Could you check a few things on this model? Use its own coordinates, in mm. A direction names the side the tool comes from. Coordinates: 2 decimals unless noted, no trailing zeros. Write each loop counter-clockwise with the first axis right and the second up, starting at its lowest first coordinate (ties: lowest second). Pieces come first, ordered by that corner, then holes. Notation, with made-up numbers: (58, 2.25) - (89, 2.25) arc R13 ccw to (89, 7.25) - close; hole circle Ø1 at (35.5, 60.25). An arc over 180 degrees is marked (long way). Answer as a JSON object with one key per item and string values. Group by question number.
1) If we section it at A-A (y = 7.62): Write out the boundary of the cut face in (x, z), plus the area to 3 significant figures.
2) If we section it at D-D (x = 13.25): Write out the boundary of the cut face in (y, z), plus the area to 3 significant figures.
3) We'd pull the mould along X, two halves only. Please class faces 1 (the cylindrical face through (5.854, 18.371, -19.108)), 2 (the flat face through (13.26, 7.51, -21.65)), 3 (the flat face through (-8, 8, -8)): released by +X, released by -X, zero draft, split by the parting line, or undercut.
4) If we section it at B-B (x = 6.35): Write out the boundary of the cut face in (y, z).
5) Will these pins go through, and if not, where does the flat tip stop? pin 1 Ø1 at (x, y) = (8.5, 3.5) entering from +Z; pin 2 Ø10 at (x, y) = (-2.5, 7) entering from +Z; pin 3 Ø6 at (y, z) = (9.5, -20.5) entering from -X.
6) On a 3-axis mill with a long thin cutter (end or side, diameter ignored), from which of +Z, -Z, +X, -X, +Y, -Y can I reach the whole of each face in a straight line? I mean faces 4 (the flat face through (3, 15.24, -13)), 5 (the flat face through (6, 8, 6.35)), 6 (the flat face through (10.5, 7.5, 0)). Say none if no direction works.
7) Please list where these lines run through material, in increasing order: line 1 along Z through (x, y) = (2.25, 5.5) (3 decimals); line 2 along Y through (x, z) = (4, -22.5); line 3 along X through (y, z) = (8.75, 1).
8) If we section it at C-C (y = 1.75): Write out the boundary of the cut face in (x, z).
```python
from build123d import *

# Parameters (mm, degrees)
BOSS_EXTRUDE1_DEPTH = 15.24
SKETCH2_R           = 3.81
BOSS_EXTRUDE2_DEPTH = 6.35
SKETCH5_R           = 3.81
BOSS_EXTRUDE3_DEPTH = 6.35


with BuildPart() as part:
    # Sketch1 → Boss-Extrude1 (new body)
    with BuildSketch(Plane(origin=(0, 0, 0), x_dir=(1, 0, 0), z_dir=(0, 1, 0))):
        Polygon((-8.980256121, 8.980256121), (0, 0), (12.7, 0), (16.220075072, 18.721954265), (10.214331376, 24.659577338), (1.769095743, 24.707745892), align=None)
    extrude(amount=BOSS_EXTRUDE1_DEPTH)

    # Sketch2 → Boss-Extrude2 (add)
    with BuildSketch(Plane.XY):
        with Locations((6.35, 7.62)):
            Circle(SKETCH2_R)
    boss_extrude2 = extrude(amount=BOSS_EXTRUDE2_DEPTH)

    # Mirror1: Boss-Extrude2 across plane
    add(boss_extrude2.mirror(Plane(origin=(0, 0, 0), x_dir=(-0.382683432, 0, 0.923879533), z_dir=(0.923879533, 0, 0.382683432))))

    # Sketch5 → Boss-Extrude3 (add)
    with BuildSketch(Plane(origin=(0, 15.24, 0), x_dir=(1, 0, 0), z_dir=(0, 1, 0))):
        with Locations((6.35, 15.330256121)):
            Circle(SKETCH5_R)
    extrude(amount=BOSS_EXTRUDE3_DEPTH)


solid = part.part
```
Here are the results:
{
 "1": {"outline": "(-11.67, -2.69) - (-7.18, -7.18) - (-8.98, -8.98) - (1.77, -24.71) - (10.21, -24.66) - (16.22, -18.72) - (12.7, 0) - (10.16, 0) - (10.16, 6.35) - (2.54, 6.35) - (2.54, 0) - (0, 0) - (-1.8, -1.8) - (-6.29, 2.69) - close", "area": "543 mm²"},
 "2": {"outline": "(0, -21.66) - (15.24, -21.66) - (15.24, -2.93) - (0, -2.93) - close", "area": "285 mm²"},
 "3": {"face 1": "split by the parting line", "face 2": "released by +X", "face 3": "undercut"},
 "4": {"outline": "(0, -24.68) - (15.24, -24.68) - (15.24, -19.14) - (21.59, -19.14) - (21.59, -11.52) - (15.24, -11.52) - (15.24, 0) - (11.43, 0) - (11.43, 6.35) - (3.81, 6.35) - (3.81, 0) - (0, 0) - close"},
 "5": {"pin 1": "stops at z = 0", "pin 2": "stops at z = 2.69", "pin 3": "stops at x = -3.16"},
 "6": {"face 4": "+Y", "face 5": "+Z, +X, -X, +Y, -Y", "face 6": "+Z"},
 "7": {"line 1": "z = -24.705 to 0", "line 2": "y = 0 to 15.24", "line 3": "x = -7.98 to -4.83, 2.71 to 9.99"},
 "8": {"outline": "(-8.98, -8.98) - (1.77, -24.71) - (10.21, -24.66) - (16.22, -18.72) - (12.7, 0) - (0, 0) - close"}
}
